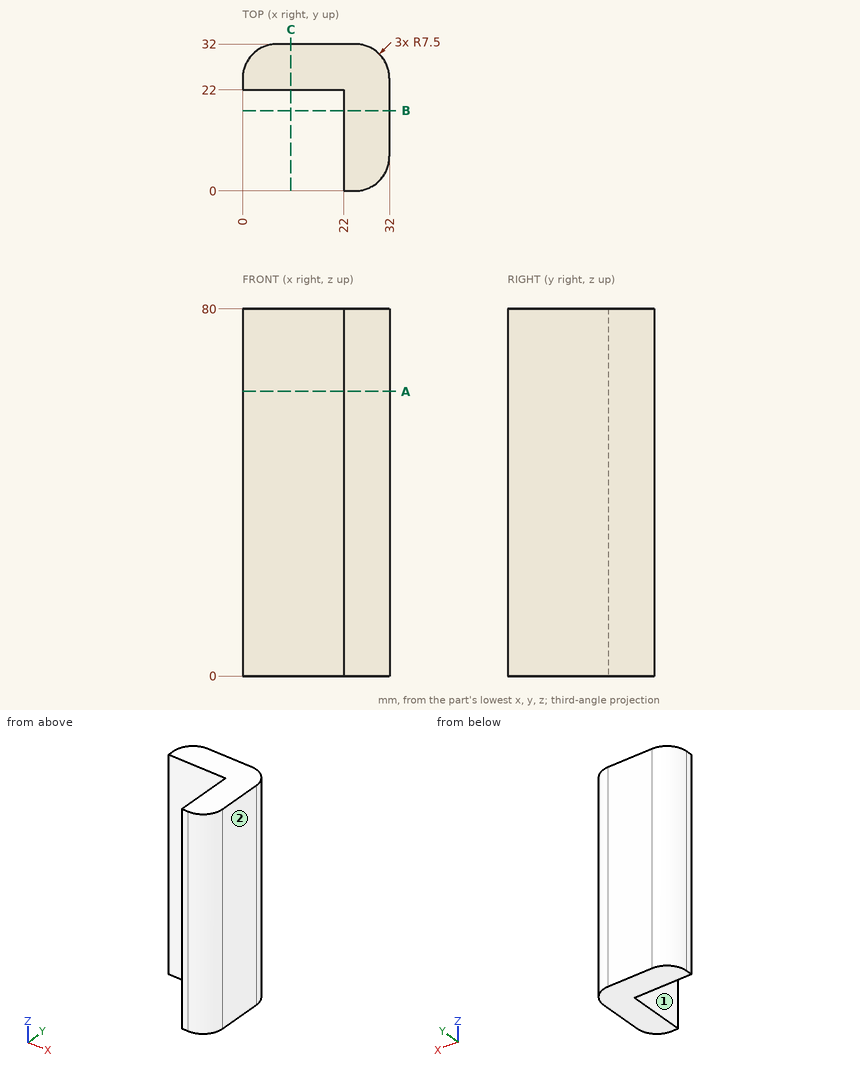
For this review, use the dimensioned drawing (mm, ordinates from the lowest corner) and the shaded views. A direction names the side the tool comes from. Coordinates: 2 decimals unless noted, no trailing zeros. Order: outer loops, then holes, each group sorted by start corner. A loop starts at its lowest first (then second) coordinate and runs counter-clockwise, first axis right, second up. Notation, with made-up numbers: (4.25, -34) -> (56.25, -34) arc R33 ccw to (56.25, -1) -> close; hole circle Ø8 at (-40, 31). An arc over 180 degrees is marked (long way). One line per item, written item: value. Start each with the question number.
Q1. For probe 1 along Y at (x, z) = (13, 11); probe 2 along Y at (x, z) = (25, 63.5), list the stretches that pass through material, from the lowest coordinate up.
Q2. Insertion check: pin 1 Ø4 at (y, z) = (9.5, 24.5) entering from -X; pin 2 Ø1 at (y, z) = (4, 24.5) entering from +X; pin 3 Ø8 at (x, z) = (15, 61.5) entering from -Y. Each pin has a flat end and moves straight along its axis. Give the tip position at first contact, or say it passes through.
Q3. Tool access review of the marked faces 1 and 2: name each direction out of +Z, -Z, +X, -X, +Y, -Y from which nothing blocks a thin tool from reaching the whole face with its end or side.
Q4. Take a section at A-A, the plane z = 62. State the section outline as (x, y) points.
Q5. Take a section at B-B, the plane y = 17.5. State the section outline as (x, z) points, then the cut area to 3 significant figures.
Values follow:
1. probe 1: y = 22 to 32
1. probe 2: y = 0.02 to 31.98
2. pin 1: stops at x = 22
2. pin 2: stops at x = 31.37
2. pin 3: stops at y = 22
3. face 1: +Z, -Z, -X, -Y
3. face 2: +Z, -Z, +X, +Y, -Y
4. outline: (0, 22) -> (22, 22) -> (22, 0) -> (24.5, 0) arc R7.5 ccw to (32, 7.5) -> (32, 24.5) arc R7.5 ccw to (24.5, 32) -> (7.5, 32) arc R7.5 ccw to (0, 24.5) -> close
5. outline: (22, 0) -> (32, 0) -> (32, 80) -> (22, 80) -> close
5. area: 800 mm2
